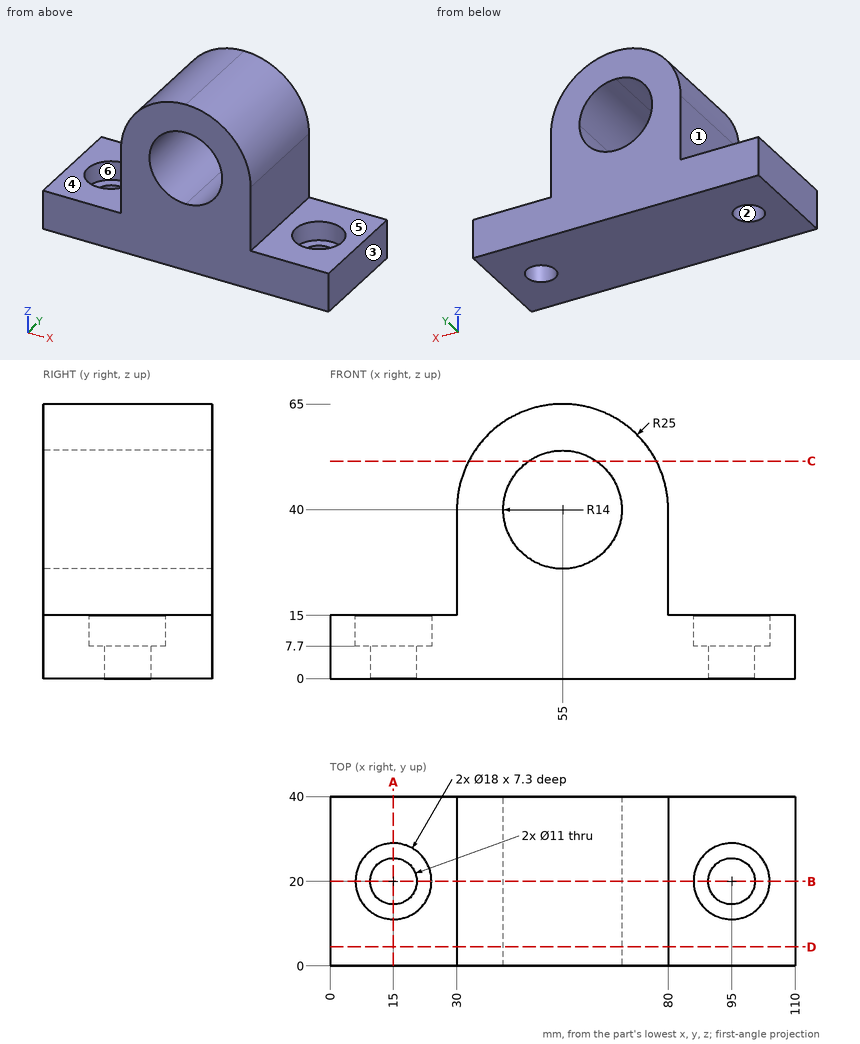
Here's the drawing with two shaded views (mm, measured from the low corner). I have some questions. A direction names the side the tool comes from. Coordinates: 2 decimals unless noted, no trailing zeros. Write each loop counter-clockwise with the first axis right and the second up, starting at its lowest first coordinate (ties: lowest second). Pieces come first, ordered by that corner, then holes. Notation, with made-up numbers: M -20.5,64.25 L 32.5,64.25 A22 ccw 32.5,103.25 Z; hole C -16.5,75 d8. An arc over 180 degrees is marked long. Answer as CSV lines item,"result". Start each with the question number.
1) For P1, Ø9, axis at x = 22.5, y = 21, coming from the +Z side; P2, Ø4, axis at x = 67, y = 28.5, coming from the +Z side; P3, Ø16, axis at x = 95, y = 20, coming from the +Z side, each with a flat end and sliding along its axis, tell me the tip position at first contact or that it passes through.
2) I want a section at A-A, the plane x = 15. Please give me the cut outline in (y, z).
3) We'd pull the mould along X, two halves only. Please class the marked faces 1, 2 and 3: +X half, -X half, draft (parallel to the pull), parting line (faces both ways), or undercut.
4) I want a section at B-B, the plane y = 20. Please give me the cut outline in (x, z).
5) For the marked faces 4, 5 and 6, which set-ups out of +Z, -Z, +X, -X, +Y, -Y let a thin tool reach every point of the face, with its end or its side?
6) Please list where these lines run through material, in increasing order: line 1 (X direction, y = 20, z = 5); line 2 (Z direction, x = 54.5, y = 15) (3 decimals); line 3 (Y direction, x = 95, z = 13). Write a range as from..to.
7) I want a section at D-D, the plane y = 4.5. Please give me the cut outline in (x, z), and give its area (3 significant figures).
8) I want a section at C-C, the plane z = 51.5. Please give me the cut outline in (x, y), and give its area (3 significant figures).
Data:
1,P1,"stops at z = 15"
1,P2,"stops at z = 62.91"
1,P3,"stops at z = 7.7"
2,outline,"M 0,0 L 14.5,0 L 14.5,7.7 L 11,7.7 L 11,15 L 0,15 Z; M 25.5,0 L 40,0 L 40,15 L 29,15 L 29,7.7 L 25.5,7.7 Z"
3,face 1,"-X half"
3,face 2,"undercut"
3,face 3,"+X half"
4,outline,"M 0,0 L 9.5,0 L 9.5,7.7 L 6,7.7 L 6,15 L 0,15 Z; M 20.5,0 L 89.5,0 L 89.5,7.7 L 86,7.7 L 86,15 L 80,15 L 80,40 A25 ccw 30,40 L 30,15 L 24,15 L 24,7.7 L 20.5,7.7 Z; M 100.5,0 L 110,0 L 110,15 L 104,15 L 104,7.7 L 100.5,7.7 Z; hole C 55,40 d28"
5,face 4,"+Z, -X, +Y, -Y"
5,face 5,"+Z, +X, +Y, -Y"
5,face 6,"+Z"
6,line 1,"x = 0..9.5, 20.5..89.5, 100.5..110"
6,line 2,"z = 0..26.009, 53.991..64.995"
6,line 3,"y = 0..11, 29..40"
7,outline,"M 0,0 L 110,0 L 110,15 L 80,15 L 80,40 A25 ccw 30,40 L 30,15 L 0,15 Z; hole C 55,40 d28"
7,area,"3,270 mm^2"
8,outline,"M 32.8,0 L 47.02,0 L 47.02,40 L 32.8,40 Z; M 62.98,0 L 77.2,0 L 77.2,40 L 62.98,40 Z"
8,area,"1,140 mm^2"
